Work out the finished part from the listing and answer in its coordinate system (mm). Round coordinates to 2 decimals unless told otherwise and drop trailing zeros. Write each loop counter-clockwise with the first axis right and the second up, starting at its lowest first coordinate (ties: lowest second). Pieces come first, ordered by that corner, then holes. Notation, with made-up numbers: (48, 39.5) -> (77, 39.5) arc R21 ccw to (77, 61.5) -> close; hole circle Ø6 at (48, 85.25). An arc over 180 degrees is marked (long way). Answer as a JSON object with one key per item and string values. Group by question number.
from build123d import *

# Parameters (mm, degrees)
BOX002_W               = 20
BOX002_H               = 7.071
BOX002_DEPTH           = 7.071
BOX002_PLACEMENT_ANGLE = 45
BOX001_W               = 20
BOX001_H               = 10
BOX001_DEPTH           = 10


with BuildPart() as cub002:
    # Box002 → Box002 (new body)
    with BuildSketch(Plane.XY):
        with Locations((10, 3.5355)):
            Rectangle(BOX002_W, BOX002_H)
    extrude(amount=BOX002_DEPTH)


with BuildPart() as cub002_1:
    # Box002 placement: moved
    add(cub002.part.moved(Location((-10, 0, 5.07))).rotate(Axis((-10, 0, 5.07), (1, 0, 0)), BOX002_PLACEMENT_ANGLE))


with BuildPart() as fusion:
    # Box001 → Box001 (new body)
    with BuildSketch(Plane(origin=(-10, -5, 0), x_dir=(1, 0, 0), z_dir=(0, 0, 1))):
        with Locations((10, 5)):
            Rectangle(BOX001_W, BOX001_H)
    extrude(amount=BOX001_DEPTH)

    # Fusion: union Cub002
    add(cub002_1.part)


solid = fusion.part
1) A cutting plane is placed at B-B on y = -0.5. Determine the outline of the cut face in (x, z).
2) Straight lines are drawn through the part: L1, parallel to Z at x = -0.75, y = 2.75; L2, parallel to Z at x = -2.25, y = 3; L3, parallel to Y at x = -0.5, z = 13.5. For each, find the intervals that lie inside material, in ascending order.
3) This flat-tipped pin is pushed along its axis until it touches: P1, Ø1, axis at x = -6, y = 3, coming from the +Z side. Where does it stop, or does it pass through?
4) A cutting plane is placed at A-A on x = 5. Determine the outline of the cut face in (y, z).
5) A cutting plane is placed at C-C on z = 14. Determine the outline of the cut face in (x, y), plus the area to 3 significant figures.
Established:
{
 "1": {"outline": "(-10, 0) -> (10, 0) -> (10, 14.57) -> (-10, 14.57) -> close"},
 "2": {"L1": "z = 0 to 12.32", "L2": "z = 0 to 12.07", "L3": "y = -1.57 to 1.57"},
 "3": {"P1": "stops at z = 12.57"},
 "4": {"outline": "(-5, 0) -> (5, 0) -> (5, 10) -> (4.93, 10) -> (5, 10.07) -> (0, 15.07) -> (-5, 10.07) -> (-4.93, 10) -> (-5, 10) -> close"},
 "5": {"outline": "(-10, -1.07) -> (10, -1.07) -> (10, 1.07) -> (-10, 1.07) -> close", "area": "42.8 mm²"}
}
